CAD build for the part. Positions are in the model's coordinates, mm. A direction names the side the tool comes from. Coordinates: 2 decimals unless noted, no trailing zeros. Loops run counter-clockwise (first coordinate to the right, second up) from the corner with the lowest first, then second, coordinate; pieces in that order, holes last. Notation, with made-up numbers: (-5, 39.5) -> (46, 39.5) arc R27 ccw to (46, 57.5) -> close; hole circle Ø5 at (77.5, 54.5). An arc over 180 degrees is marked (long way). Write each question's results on one line, items separated by ' | '.
```python
from build123d import *

# Parameters (mm, degrees)
F0_R     = 11
F1_DEPTH = 1.5
F2_R     = 5
F3_DEPTH = 0.5
F4_R     = 4
F5_DEPTH = 2
F6_R     = 0.5


# Not quite as in the source:
# - a fillet or chamfer that OpenCascade refuses, or shapes differently, is made with other operations: its cross-section is extruded or revolved along the edge and cut away or added


with BuildPart() as f1:
    # F0 (on Top) → F1 (new body)
    with BuildSketch(Plane.XY):
        Circle(F0_R)
    extrude(amount=F1_DEPTH)

    # F2 (on face) → F3 (join)
    with BuildSketch(Plane.XY.offset(1.5)):
        Circle(F2_R)
    extrude(amount=F3_DEPTH)

    # F4 (on face) → F5 (join)
    with BuildSketch(Plane.XY.offset(2)):
        Circle(F4_R)
    extrude(amount=F5_DEPTH)

    # F6
    f6_edges = [f1.edges().sort_by_distance(p)[0] for p in [
        (-4, 0, 4),
    ]]
    fillet(f6_edges, radius=F6_R)

    # F7: fillet of radius 2 on 1 edges, made by hand

    # F7_s1 → F7_t2 (revolve, cut)
    with BuildSketch(Plane.XZ):
        with BuildLine():
            ThreePointArc((9.0635083269, 1.5), (10.2882531983, 1.0811388301), (11, 0))
            Line((11, 0), (11, 1.5))
            Line((11, 1.5), (9.0635083269, 1.5))
        make_face()
    revolve(axis=Axis((0, 0, 1.5), (0, 0, 1)), mode=Mode.SUBTRACT)


solid = f1.part
```
Q1. Wall check: L1, parallel to Z at x = -1.25, y = 8.25; L2, parallel to Z at x = 4.5, y = 0.75; L3, parallel to X at y = 4.75, z = 0.75. Give the ranges that are in metal, low to high. Write a range as from..to.
Results are:
L1: 0..1.5 | L2: 0..2 | L3: -9.5..9.5
Q2. Which spindle directions (+Z, -Z, +X, -X, +Y, -Y) get a long thin tool onto all of the face, cutting with end or side? Do faces 1 (the cylindrical face through (-1.08, -4.88, 1.75)), 2 (the flat face through (0, 0, 0)). Say none if no direction does.
Results are:
face 1: +Z | face 2: -Z, +X, -X, +Y, -Y
Q3. Cut at C-C on z = 2.3. Write the cut outline in (x, y), and give its area (3 significant figures).
Results are:
outline: circle Ø8 at (0, 0) | area: 50.3 mm^2
Q4. Cut at D-D on z = 1.2. Write the cut outline in (x, y), and give its area (3 significant figures).
Results are:
outline: circle Ø20.23 at (0, 0) | area: 322 mm^2
Q5. Drop flat-ended pins along their axis: pin 1 (10 mm diameter, centred on x = 5, y = -6, fed in from -Z); pin 2 (1.5 mm diameter, centred on x = -0.5, z = 1, fed in from +Y); pin 3 (1.5 mm diameter, centred on x = -7.5, z = 2.5, fed in from +Y); pin 4 (1.5 mm diameter, centred on y = 7, z = 0.5, fed in from +X). Give the stop position or say it passes through.
Results are:
pin 1: z = 0 | pin 2: y = 10.91 | pin 3: through | pin 4: x = 8.94
Q6. Cut at A-A on x = 0. Write the cut outline in (y, z), and give its area (3 significant figures).
Results are:
outline: (-11, 0) -> (11, 0) arc R2 ccw to (9.06, 1.5) -> (5, 1.5) -> (5, 2) -> (4, 2) -> (4, 3.5) arc R0.5 ccw to (3.5, 4) -> (-3.5, 4) arc R0.5 ccw to (-4, 3.5) -> (-4, 2) -> (-5, 2) -> (-5, 1.5) -> (-9.06, 1.5) arc R2 ccw to start | area: 52.4 mm^2
